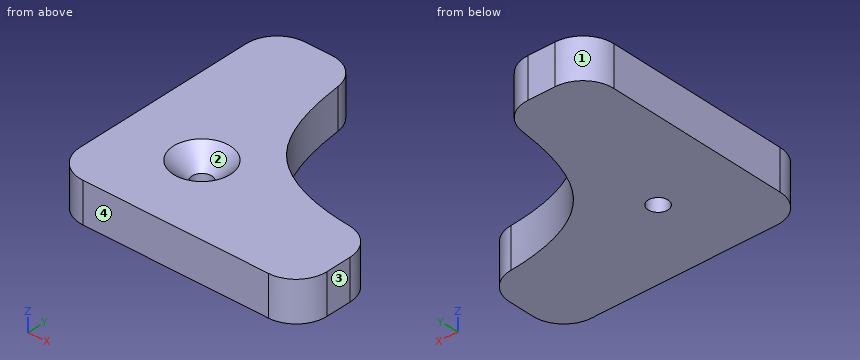
```python
from build123d import *

# Parameters (mm, degrees)
F1_R     = 1.6
F2_DEPTH = 6.5
F3_SIZE  = 3
F4_R     = 5


with BuildPart() as f2:
    # F1 (on Top) → F2 (new body)
    with BuildSketch(Plane.XY):
        with BuildLine():
            Line((-6, 20), (-20, 20))
            Line((-20, 20), (-20, -20))
            Line((-20, -20), (20, -20))
            Line((20, -20), (20, -6))
            add(Edge.make_bspline(
                [(-6, 20), (-5.4739157377, 12.0071208998), (-3.301555689, -2.9531264796), (12.0770271157, -6.1008679405), (20, -6)],
                knots=[0, 0, 0, 0, 0.5, 1, 1, 1, 1], degree=3))
        make_face()
        with Locations((-7.2231281083, -7.2231281083)):
            Circle(F1_R, mode=Mode.SUBTRACT)
    extrude(amount=F2_DEPTH)

    # F3
    f3_edges = [f2.edges().sort_by_distance(p)[0] for p in [
        (-8.823128, -7.223128, 6.5),
    ]]
    chamfer(f3_edges, length=F3_SIZE)

    # F4
    f4_edges = [f2.edges().sort_by_distance(p)[0] for p in [
        (-20, -20, 3.25),
        (20, -20, 3.25),
        (20, -6, 3.25),
        (-20, 20, 3.25),
        (-6, 20, 3.25),
    ]]
    fillet(f4_edges, radius=F4_R)


solid = f2.part
```
Source: CAD feature listing. Evaluate the final solid. Frame: model axes, mm. Face numbers are marked on the shaded views. Round coordinates to 2 decimals unless told otherwise and drop trailing zeros. Loops run counter-clockwise (first coordinate to the right, second up) from the corner with the lowest first, then second, coordinate; pieces in that order, holes last.
1. Contact query for a flat-ended pin moving along its axis: pin 1 (1 mm diameter, centred on x = -1.5, z = 1, fed in from +Y). Output: stop coordinate, or through.
2. Section query A-A on x = -17. Output: boundary loops of the cut face in (y, z).
3. Mould query, pull axis X, two halves, no side actions, for the marked faces 1, 2, 3 and 4. Classes: released by +X, released by -X, zero draft, split by the parting line, or undercut.
4. Ray query, L1, parallel to Y at x = -7, z = 3.75; L2, parallel to Y at x = 14.5, z = 3; L3, parallel to Y at x = -1, z = 0.5. Return the intervals inside material, ascending.
Answers below:
1. pin 1: stops at y = 2.61
2. outline: (-19.58, 0) - (19.58, 0) - (19.58, 6.5) - (-19.58, 6.5) - close
3. face 1: released by -X
3. face 2: undercut
3. face 3: released by +X
3. face 4: zero draft
4. L1: y = -20 to -9.06, -5.39 to 18.48
4. L2: y = -20 to -5.78
4. L3: y = -20 to 1.15
